from build123d import *

# Parameters (mm, degrees)
F0_W     = 368.3
F0_H     = 12.7
F0_W_2   = 19.05
F0_H_2   = 33.02
F1_DEPTH = 19.05
F2_DEPTH = 6.35
F3_DEPTH = 6.35


with BuildPart() as f1:
    # F0 (on Right) → F1 (new body)
    with BuildSketch(Plane.YZ):
        with Locations((-24.839816, 101.602047)):
            Rectangle(F0_W, F0_H)
        Polygon((159.310184, 95.252047), (-208.989816, 95.252047), (-208.989816, 74.932047), (-208.989816, 41.912047), (-208.989816, 8.892047), (-208.989816, -24.127953), (-208.989816, -44.447953), (159.310184, -44.447953), (159.310184, -24.127953), (159.310184, 8.892047), (159.310184, 41.912047), (159.310184, 74.932047), align=None)
        with Locations((-218.514816, 58.422047)):
            Rectangle(F0_W_2, F0_H_2)
        with Locations((168.835184, 58.422047)):
            Rectangle(F0_W_2, F0_H_2)
        with Locations((-218.514816, -7.617953)):
            Rectangle(F0_W_2, F0_H_2)
        with Locations((168.835184, -7.617953)):
            Rectangle(F0_W_2, F0_H_2)
        with Locations((-24.839816, -50.797953)):
            Rectangle(F0_W, F0_H)
    extrude(amount=F1_DEPTH)

    # F0 (on Right) → F2 (cut)
    with BuildSketch(Plane.YZ):
        with Locations((-24.839816, 101.602047)):
            Rectangle(F0_W, F0_H)
    extrude(amount=F2_DEPTH, mode=Mode.SUBTRACT)

    # F0 (on Right) → F3 (cut)
    with BuildSketch(Plane.YZ):
        with Locations((-24.839816, -50.797953)):
            Rectangle(F0_W, F0_H)
    extrude(amount=F3_DEPTH, mode=Mode.SUBTRACT)


solid = f1.part
Input: part model. Units: mm. Frame: model coordinates. A direction names the side the tool comes from. Coordinates: 2 decimals unless noted, no trailing zeros. Order: outer loops, then holes, each group sorted by start corner. A loop starts at its lowest first (then second) coordinate and runs counter-clockwise, first axis right, second up. Notation, with made-up numbers: M -7,-6.75 L -1,-6.75 A18 cw -1,5.25 Z; hole C 51,88 d1. An arc over 180 degrees is marked long. Answer in a Markdown table with one row per item.
(1) Section query A-A, the plane x = 13.25. Output: boundary loops of the cut face in (y, z).
Numbers:
| item | result |
|---|---|
| outline | M -228.04,-24.13 L -208.99,-24.13 L -208.99,-57.15 L 159.31,-57.15 L 159.31,-24.13 L 178.36,-24.13 L 178.36,8.89 L 159.31,8.89 L 159.31,41.91 L 178.36,41.91 L 178.36,74.93 L 159.31,74.93 L 159.31,107.95 L -208.99,107.95 L -208.99,74.93 L -228.04,74.93 L -228.04,41.91 L -208.99,41.91 L -208.99,8.89 L -228.04,8.89 Z |
(2) Material intervals for line 1 (Y direction, x = 16.75, z = 99); line 2 (Z direction, x = 2, y = -65.5); line 3 (X direction, y = -84.5, z = -47.5), sorted ascending. Write a range as [from, to].
Numbers:
| item | result |
|---|---|
| line 1 | y = [-208.99, 159.31] |
| line 2 | z = [-44.45, 95.25] |
| line 3 | x = [6.35, 19.05] |
(3) Contact query for flat-ended pins moving along their axis: pin 1 Ø1 at (x, z) = (13, 22.5) entering from -Y; pin 2 Ø14 at (y, z) = (-44.5, -48.5) entering from -X; pin 3 Ø5.5 at (x, z) = (7, -45.5) entering from +Y; pin 4 Ø9.5 at (x, y) = (13, 170) entering from +Z. Output: stop coordinate, or through.
Numbers:
| item | result |
|---|---|
| pin 1 | stops at y = -208.99 |
| pin 2 | stops at x = 0 |
| pin 3 | stops at y = 159.31 |
| pin 4 | stops at z = 74.93 |
(4) Access query for faces 1 (the flat face through (9, -219, 8.892)), 2 (the flat face through (9, 169, 74.932)), 3 (the flat face through (12, -208.99, 92)). Directions: +Z, -Z, +X, -X, +Y, -Y. A direction counts if a zero-diameter tool reaches every point of the face in a straight line with its end or side. Return the directions, or none.
Numbers:
| item | result |
|---|---|
| face 1 | +X, -X, -Y |
| face 2 | +Z, +X, -X, +Y |
| face 3 | +Z, +X, -X, -Y |
(5) Section query C-C, the plane z = -32. Output: boundary loops of the cut face in (x, y).
Numbers:
| item | result |
|---|---|
| outline | M 0,-208.99 L 19.05,-208.99 L 19.05,159.31 L 0,159.31 Z |
(6) Draft query along Z for faces 4 (the flat face through (9, -219, 74.932)), 5 (the flat face through (9, 169, -24.128)), 6 (the flat face through (9, -219, 41.912)), 7 (the flat face through (9, -228.04, -8)). Return one class per face: pulls with the +Z half, pulls with the -Z half, needs draft (parallel to the pull), parting line crosses it, or undercut.
Numbers:
| item | result |
|---|---|
| face 4 | pulls with the +Z half |
| face 5 | pulls with the -Z half |
| face 6 | undercut |
| face 7 | needs draft |
(7) Section query B-B, the plane y = -37.5. Output: boundary loops of the cut face in (x, z), plus the area to 3 significant figures.
Numbers:
| item | result |
|---|---|
| outline | M 0,-44.45 L 6.35,-44.45 L 6.35,-57.15 L 19.05,-57.15 L 19.05,107.95 L 6.35,107.95 L 6.35,95.25 L 0,95.25 Z |
| area | 2,980 mm^2 |
